from build123d import *

# Parameters (mm, degrees)
SKETCH1_W                     = 80
SKETCH1_H                     = 20
BOSS_EXTRUDE1_DEPTH           = 19.85
CUT_EXTRUDE1_REACH            = 86.818
SKETCH2_R                     = 3.1
CUT_EXTRUDE2_REACH            = 86.818
SKETCH3_R                     = 5
FILLET1_R                     = 1
CSK_FOR_M6_SFHCS1_D           = 6.6
CSK_FOR_M6_SFHCS1_DEPTH       = 19.85
CSK_FOR_M6_SFHCS1_CSINK_D     = 13.44
CSK_FOR_M6_SFHCS1_CSINK_ANGLE = 90
M3X0_5_TAPPED_HOLE1_REACH     = 86.818
M3X0_5_TAPPED_HOLE1_BORE_R    = 1.25


with BuildPart() as part:
    # Sketch1 → Boss-Extrude1 (new body)
    with BuildSketch(Plane(origin=(0, 0, 0), x_dir=(1, 0, 0), z_dir=(0, 1, 0))):
        with Locations((40, 10)):
            Rectangle(SKETCH1_W, SKETCH1_H)
    extrude(amount=BOSS_EXTRUDE1_DEPTH)

    # Sketch2 → Cut-Extrude1 (cut, up to next)
    with BuildSketch(Plane(origin=(0, 19.85, 0), x_dir=(1, 0, 0), z_dir=(0, 1, 0)), mode=Mode.PRIVATE) as cut_extrude1_sk1:
        with Locations(Location((20, 10, 0), (0, 0, 270))):
            Circle(SKETCH2_R)
    cut_extrude1_tool1 = extrude(cut_extrude1_sk1.sketch, amount=-CUT_EXTRUDE1_REACH, mode=Mode.PRIVATE) & part.part
    # Sketch2 → Cut-Extrude1 (cut, up to next)
    with BuildSketch(Plane(origin=(0, 19.85, 0), x_dir=(1, 0, 0), z_dir=(0, 1, 0)), mode=Mode.PRIVATE) as cut_extrude1_sk2:
        with Locations(Location((60, 10, 0), (0, 0, 270))):
            Circle(SKETCH2_R)
    cut_extrude1_tool2 = extrude(cut_extrude1_sk2.sketch, amount=-CUT_EXTRUDE1_REACH, mode=Mode.PRIVATE) & part.part
    add(cut_extrude1_tool1.solids().sort_by_distance((20, 19.85, -10))[0], mode=Mode.SUBTRACT)
    add(cut_extrude1_tool2.solids().sort_by_distance((60, 19.85, -10))[0], mode=Mode.SUBTRACT)

    # Sketch3 → Cut-Extrude2 (cut, up to next)
    with BuildSketch(Plane.XY, mode=Mode.PRIVATE) as cut_extrude2_sk1:
        with Locations((7.5, 11.85)):
            Circle(SKETCH3_R)
    cut_extrude2_tool1 = extrude(cut_extrude2_sk1.sketch, amount=-CUT_EXTRUDE2_REACH, mode=Mode.PRIVATE) & part.part
    # Sketch3 → Cut-Extrude2 (cut, up to next)
    with BuildSketch(Plane.XY, mode=Mode.PRIVATE) as cut_extrude2_sk2:
        with Locations((72.5, 11.85)):
            Circle(SKETCH3_R)
    cut_extrude2_tool2 = extrude(cut_extrude2_sk2.sketch, amount=-CUT_EXTRUDE2_REACH, mode=Mode.PRIVATE) & part.part
    # Sketch3 → Cut-Extrude2 (cut, up to next)
    with BuildSketch(Plane.XY, mode=Mode.PRIVATE) as cut_extrude2_sk3:
        with Locations((40, 11.85)):
            Circle(SKETCH3_R)
    cut_extrude2_tool3 = extrude(cut_extrude2_sk3.sketch, amount=-CUT_EXTRUDE2_REACH, mode=Mode.PRIVATE) & part.part
    add(cut_extrude2_tool1.solids().sort_by_distance((7.5, 11.85, 0))[0], mode=Mode.SUBTRACT)
    add(cut_extrude2_tool2.solids().sort_by_distance((72.5, 11.85, 0))[0], mode=Mode.SUBTRACT)
    add(cut_extrude2_tool3.solids().sort_by_distance((40, 11.85, 0))[0], mode=Mode.SUBTRACT)

    # Fillet1
    fillet1_edges = [part.edges().sort_by_distance(p)[0] for p in [
        (80, 19.85, -10),
        (40, 19.85, -20),
        (0, 19.85, -10),
        (40, 0, -20),
        (80, 0, -10),
        (40, 0, 0),
        (0, 0, -10),
        (40, 19.85, 0),
        (0, 9.925, -20),
        (80, 9.925, -20),
        (80, 9.925, 0),
        (0, 9.925, 0),
    ]]
    fillet(fillet1_edges, radius=FILLET1_R)

    # CSK for M6 SFHCS1
    with Locations(Plane(origin=(0, 19.85, 0), x_dir=(1, 0, 0), z_dir=(0, 1, 0))):
        with Locations((60, 10), (20, 10)):
            CounterSinkHole(CSK_FOR_M6_SFHCS1_D / 2, CSK_FOR_M6_SFHCS1_CSINK_D / 2, depth=CSK_FOR_M6_SFHCS1_DEPTH, counter_sink_angle=CSK_FOR_M6_SFHCS1_CSINK_ANGLE)

    # M3x0.5 Tapped Hole1 bore → M3x0.5 Tapped Hole1 (cut, up to next)
    with BuildSketch(Plane(origin=(0, 19.85, 0), x_dir=(1, 0, 0), z_dir=(0, 1, 0)), mode=Mode.PRIVATE) as m3x0_5_tapped_hole1_sk1:
        with Locations((7.5, 10)):
            Circle(M3X0_5_TAPPED_HOLE1_BORE_R)
    m3x0_5_tapped_hole1_tool1 = extrude(m3x0_5_tapped_hole1_sk1.sketch, amount=-M3X0_5_TAPPED_HOLE1_REACH, mode=Mode.PRIVATE) & part.part
    # M3x0.5 Tapped Hole1 bore → M3x0.5 Tapped Hole1 (cut, up to next)
    with BuildSketch(Plane(origin=(0, 19.85, 0), x_dir=(1, 0, 0), z_dir=(0, 1, 0)), mode=Mode.PRIVATE) as m3x0_5_tapped_hole1_sk2:
        with Locations((40, 10)):
            Circle(M3X0_5_TAPPED_HOLE1_BORE_R)
    m3x0_5_tapped_hole1_tool2 = extrude(m3x0_5_tapped_hole1_sk2.sketch, amount=-M3X0_5_TAPPED_HOLE1_REACH, mode=Mode.PRIVATE) & part.part
    # M3x0.5 Tapped Hole1 bore → M3x0.5 Tapped Hole1 (cut, up to next)
    with BuildSketch(Plane(origin=(0, 19.85, 0), x_dir=(1, 0, 0), z_dir=(0, 1, 0)), mode=Mode.PRIVATE) as m3x0_5_tapped_hole1_sk3:
        with Locations((72.5, 10)):
            Circle(M3X0_5_TAPPED_HOLE1_BORE_R)
    m3x0_5_tapped_hole1_tool3 = extrude(m3x0_5_tapped_hole1_sk3.sketch, amount=-M3X0_5_TAPPED_HOLE1_REACH, mode=Mode.PRIVATE) & part.part
    add(m3x0_5_tapped_hole1_tool1.solids().sort_by_distance((7.5, 19.85, -10))[0], mode=Mode.SUBTRACT)
    add(m3x0_5_tapped_hole1_tool2.solids().sort_by_distance((40, 19.85, -10))[0], mode=Mode.SUBTRACT)
    add(m3x0_5_tapped_hole1_tool3.solids().sort_by_distance((72.5, 19.85, -10))[0], mode=Mode.SUBTRACT)


solid = part.part
The listing builds one solid part. Answer for the finished solid, in the listing's coordinates (mm). A direction names the side the tool comes from. Coordinates: 2 decimals unless noted, no trailing zeros. Write each loop counter-clockwise with the first axis right and the second up, starting at its lowest first coordinate (ties: lowest second). Pieces come first, ordered by that corner, then holes. Notation, with made-up numbers: (52.25, -6) - (71.25, -6) arc R15 ccw to (71.25, 19) - close; hole circle Ø8 at (-16.75, -35.75). An arc over 180 degrees is marked (long way). Put each result on its own line as item: value.
1. The part is cut by section B-B on x = 7.5. Give the vertices of the cut face in (y, z).
Answer sheet:
outline: (0, -19) arc R1 ccw to (1, -20) - (6.85, -20) - (6.85, 0) - (1, 0) arc R1 ccw to (0, -1) - close; (16.85, -20) - (18.85, -20) arc R1 ccw to (19.85, -19) - (19.85, -11.25) - (16.85, -11.25) - close; (16.85, -8.75) - (19.85, -8.75) - (19.85, -1) arc R1 ccw to (18.85, 0) - (16.85, 0) - close
2. The part is cut by section C-C on y = 4.5. Give the vertices of the cut face in (x, z).
Answer sheet:
outline: (0, -19) arc R1 ccw to (1, -20) - (79, -20) arc R1 ccw to (80, -19) - (80, -1) arc R1 ccw to (79, 0) - (1, 0) arc R1 ccw to (0, -1) - close; hole circle Ø6.6 at (20, -10); hole circle Ø6.6 at (60, -10)
3. The part is cut by section A-A on y = 13.25. Give the vertices of the cut face in (x, z).
Answer sheet:
outline: (0, -19) arc R1 ccw to (1, -20) - (2.7, -20) - (2.7, 0) - (1, 0) arc R1 ccw to (0, -1) - close; (12.3, -20) - (35.2, -20) - (35.2, 0) - (12.3, 0) - close; (44.8, -20) - (67.7, -20) - (67.7, 0) - (44.8, 0) - close; (77.3, -20) - (79, -20) arc R1 ccw to (80, -19) - (80, -1) arc R1 ccw to (79, 0) - (77.3, 0) - close; hole circle Ø6.6 at (20, -10); hole circle Ø6.6 at (60, -10)
4. Find the intervals of material crossed by line 1 along X through (y, z) = (5.5, -10); line 2 along X through (y, z) = (12, -15); line 3 along Z through (x, y) = (60, 7.25), in increasing order. Write a range as from..to.
Answer sheet:
line 1: x = 0..16.7, 23.3..56.7, 63.3..80
line 2: x = 0..2.5, 12.5..35, 45..67.5, 77.5..80
line 3: z = -20..-13.3, -6.7..0
5. Determine the mould class of faces 1 (the face through (39, 6, -20)), 2 (the face through (18.401, 16.596, -6.925)), 3 (the face through (74.807, 7.414, -9.86)) for opening direction Y: pulls with the +Y half, pulls with the -Y half, needs draft (parallel to the pull), parting line crosses it, or undercut.
Answer sheet:
face 1: needs draft
face 2: pulls with the +Y half
face 3: undercut
6. The part is cut by section D-D on z = -10. State how many separate pieces and enclosed holes the cut face has, plus the area to 3 significant figures.
Answer sheet:
separate pieces: 3
enclosed holes: 0
area: 1,040 mm^2
7. A tool of negligible diameter and unlimited length cuts with its end or side. For faces 4 (the face through (73.69, 18.29, -10.38)), 5 (the face through (18.48, 8.1, -7.07)), from which of +Z, -Z, +X, -X, +Y, -Y can it reach the whole face along a straight path? Write none if from no direction.
Answer sheet:
face 4: +Y
face 5: +Y, -Y
